Can you work these out from the model? Positions are in its coordinate system, mm. Give positions to 0.01 mm unless a question says otherwise; leave off trailing zeros. Loops run counter-clockwise (first coordinate to the right, second up) from the corner with the lowest first, then second, coordinate; pieces in that order, holes last. Notation, with made-up numbers: M 34.5,22.25 L 41.5,22.25 A3 ccw 41.5,26.25 Z; hole C 29.25,-40 d8. An arc over 180 degrees is marked long. Put each result on its own line as item: value. Start each with the question number.
1) Imagine slicing it at D-D (z = 4.2). State how many separate pieces and enclosed holes the cut face has, then the cut area to 3 significant figures.
2) Imagine slicing it at B-B (y = 0). Write out the boundary of the cut face in (x, z).
3) Imagine slicing it at A-A (x = 0). Write out the boundary of the cut face in (y, z).
4) For P1, Ø2, axis at y = -57, z = 3.5, coming from the +X side; P2, Ø3, axis at x = -16.5, z = 3, coming from the +Y side; P3, Ø2, axis at y = -55, z = 1.5, coming from the +X side, each with a flat end and sliding along its axis, tell me the tip position at first contact or that it passes through.
5) Imagine slicing it at C-C (x = -20). Write out the boundary of the cut face in (y, z).
6) Please list where these lines run through material, in increasing order: line 1 along Y through (x, z) = (0, 1.5); line 2 along Y through (x, z) = (1, 5.45); line 3 along X through (y, z) = (1, 0.75). Write a range as from..to.
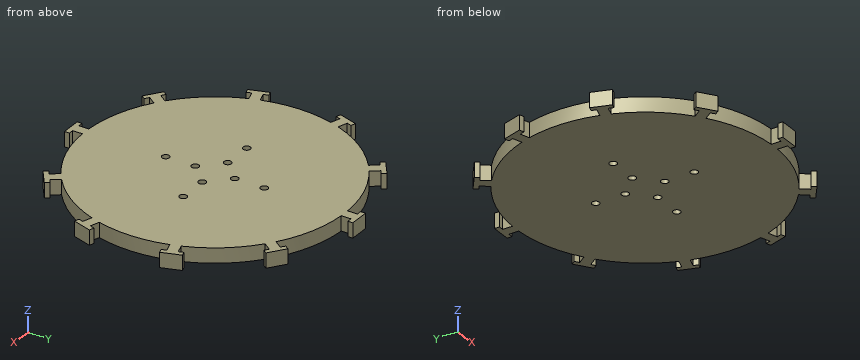
from build123d import *
from build123d.topology import SkipClean

# Parameters (mm, degrees)
SKETCH1_R           = 52.5
BOSS_EXTRUDE1_DEPTH = 2
BOSS_EXTRUDE2_DEPTH = 6
CIRPATTERN1_COUNT   = 10
SKETCH4_R           = 1.5
CUT_EXTRUDE2_DEPTH  = 10
SKETCH7_R           = 1.5
CUT_EXTRUDE3_DEPTH  = 10


with BuildPart() as part:
    # Sketch1 → Boss-Extrude1 (new body)
    with BuildSketch(Plane.XY):
        Circle(SKETCH1_R)
    extrude(amount=BOSS_EXTRUDE1_DEPTH)

    # Sketch6 → Boss-Extrude2 (add)
    with SkipClean():  # the faces are left unmerged after this step: merging them gives an invalid solid
        with BuildSketch(Plane.XY):
            with BuildLine():
                Line((-2, 52.46189093), (-2, 56.46189093))
                Line((-2, 56.46189093), (-4, 56.46189093))
                Line((-4, 56.46189093), (-4, 58.46189093))
                Line((-4, 58.46189093), (4, 58.46189093))
                Line((4, 58.46189093), (4, 56.46189093))
                Line((4, 56.46189093), (2, 56.46189093))
                Line((2, 56.46189093), (2, 52.46189093))
                ThreePointArc((2, 52.46189093), (0, -52.5), (-2, 52.46189093))
            make_face()
        boss_extrude2 = extrude(amount=BOSS_EXTRUDE2_DEPTH)

    # CirPattern1: Boss-Extrude2 ×10 about axis
    cirpattern1_axis = Axis((0, 0, 0), (0, 0, 1))
    for i in range(1, CIRPATTERN1_COUNT):
        add(boss_extrude2.rotate(cirpattern1_axis, i * 360 / CIRPATTERN1_COUNT))

    # Sketch4 → Cut-Extrude2 (cut, symmetric)
    with BuildSketch(Plane.XY.offset(2)):
        with Locations((0, 8)):
            Circle(SKETCH4_R)
        with Locations((8, 0)):
            Circle(SKETCH4_R)
        with Locations((0, -8)):
            Circle(SKETCH4_R)
        with Locations((-8, 0)):
            Circle(SKETCH4_R)
    extrude(amount=CUT_EXTRUDE2_DEPTH, both=True, mode=Mode.SUBTRACT)

    # Sketch7 → Cut-Extrude3 (cut, symmetric)
    with BuildSketch(Plane.XY.offset(6)):
        with Locations((0, 20)):
            Circle(SKETCH7_R)
        with Locations((20, 0)):
            Circle(SKETCH7_R)
        with Locations((0, -20)):
            Circle(SKETCH7_R)
        with Locations((-20, 0)):
            Circle(SKETCH7_R)
    extrude(amount=CUT_EXTRUDE3_DEPTH, both=True, mode=Mode.SUBTRACT)


solid = part.part
Recorded:
1. separate pieces: 1
1. enclosed holes: 8
1. area: 8,920 mm²
2. outline: M -52.5,0 L -21.5,0 L -21.5,6 L -52.5,6 Z; M -18.5,0 L -9.5,0 L -9.5,6 L -18.5,6 Z; M -6.5,0 L 6.5,0 L 6.5,6 L -6.5,6 Z; M 9.5,0 L 18.5,0 L 18.5,6 L 9.5,6 Z; M 21.5,0 L 52.5,0 L 52.5,6 L 21.5,6 Z
3. outline: M -58.46,0 L -21.5,0 L -21.5,6 L -58.46,6 Z; M -18.5,0 L -9.5,0 L -9.5,6 L -18.5,6 Z; M -6.5,0 L 6.5,0 L 6.5,6 L -6.5,6 Z; M 9.5,0 L 18.5,0 L 18.5,6 L 9.5,6 Z; M 21.5,0 L 58.46,0 L 58.46,6 L 21.5,6 Z
4. P1: x = 4
4. P2: y = 50.31
4. P3: x = 2
5. outline: M -48.54,0 L -1.5,0 L -1.5,6 L -48.54,6 Z; M 1.5,0 L 48.54,0 L 48.54,6 L 1.5,6 Z
6. line 1: -58.46..-21.5, -18.5..-9.5, -6.5..6.5, 9.5..18.5, 21.5..58.46
6. line 2: -58.46..-21.12, -18.88..-9.12, -6.88..6.88, 9.12..18.88, 21.12..58.46
6. line 3: -52.49..-21.12, -18.88..-9.12, -6.88..6.88, 9.12..18.88, 21.12..52.49
